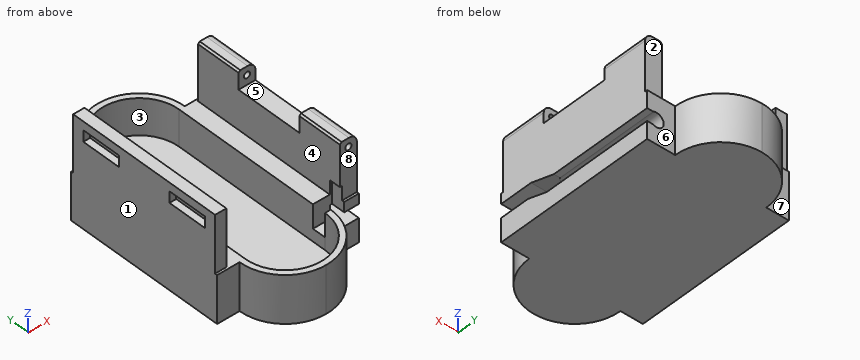
```python
from build123d import *

# Parameters (mm, degrees)
SKETCH_1_W           = 24.2
SKETCH_1_H           = 45
EXTRUDE_1_DEPTH      = 18.5
CUT_EXTRUDE_1_DEPTH  = 10.1
CUT_EXTRUDE_2_DEPTH  = 6.4
CUT_EXTRUDE_3_DEPTH  = 9.4
CUT_EXTRUDE_4_DEPTH  = 9.4
SKETCH_6_W           = 2.4
SKETCH_6_H           = 2.4
CUT_EXTRUDE_5_DEPTH  = 6.4
SKETCH_8_W           = 3.4
SKETCH_8_H           = 2.4
CUT_EXTRUDE_7_DEPTH  = 2
SKETCH_9_W           = 2.5
SKETCH_9_H           = 2
CUT_EXTRUDE_8_DEPTH  = 0.4
SKETCH_12_W          = 18.5
SKETCH_12_H          = 26.4
EXTRUDE_2_DEPTH      = 1
SKETCH_13_R          = 1.25
CUT_EXTRUDE_10_DEPTH = 26.4
SKETCH_14_W          = 2.2
SKETCH_14_H          = 26.4
CUT_EXTRUDE_11_DEPTH = 1.5
CUT_EXTRUDE_13_DEPTH = 2.95
SKETCH_19_W          = 10.1
SKETCH_19_H          = 2
EXTRUDE_3_DEPTH      = 1
SKETCH_20_W          = 1.8
SKETCH_20_H          = 2.4
EXTRUDE_4_DEPTH      = 1
SKETCH_21_W          = 1
SKETCH_21_H          = 10.1
CUT_EXTRUDE_14_DEPTH = 0.4
SKETCH_22_W          = 4.2
SKETCH_22_H          = 2.4
EXTRUDE_5_DEPTH      = 1
EXTRUDE_6_DEPTH      = 2.95
SKETCH_25_W          = 3
SKETCH_25_H          = 12
CUT_EXTRUDE_15_DEPTH = 3.2
SKETCH_26_R          = 0.55
CUT_EXTRUDE_16_DEPTH = 26
FILLET_1_R           = 1.4
SKETCH_27_W          = 2
SKETCH_27_H          = 7
CUT_EXTRUDE_17_DEPTH = 1.2
CHAMFER_1_SIZE       = 0.3


with BuildPart() as part:
    # 草图1 → 凸台-拉伸1 (new body)
    with BuildSketch(Plane.XY):
        with Locations((12.1, -22.5)):
            Rectangle(SKETCH_1_W, SKETCH_1_H)
    extrude(amount=EXTRUDE_1_DEPTH)

    # 草图2 → 切除-拉伸1 (cut)
    with BuildSketch(Plane.XY.offset(18.5)):
        Polygon((0, 0), (0, -8.5), (2, -8.5), (2, -36.5), (0, -36.5), (0, -45), (24.2, -45), (24.2, -36.5), (22.2, -36.5), (22.2, -8.5), (24.2, -8.5), (24.2, 0), align=None)
    extrude(amount=-CUT_EXTRUDE_1_DEPTH, mode=Mode.SUBTRACT)

    # 草图3 → 切除-拉伸2 (cut)
    with BuildSketch(Plane.XY.offset(8.4)):
        with BuildLine():
            Line((5, -8.1), (5, -36.9))
            ThreePointArc((5, -36.9), (12.1, -44), (19.2, -36.9))
            Line((19.2, -36.9), (19.2, -8.1))
            ThreePointArc((19.2, -8.1), (12.1, -1), (5, -8.1))
        make_face()
    extrude(amount=-CUT_EXTRUDE_2_DEPTH, mode=Mode.SUBTRACT)

    # 草图4 → 切除-拉伸3 (cut, through all)
    with BuildSketch(Plane.XY.offset(8.4)):
        with BuildLine():
            Line((4, -8.1), (0, -8.1))
            Line((0, -8.1), (0, 0))
            Line((0, 0), (12.1, 0))
            ThreePointArc((12.1, 0), (6.372435072, -2.372435072), (4, -8.1))
        make_face()
        with BuildLine():
            Line((4, -36.9), (0, -36.9))
            Line((0, -36.9), (0, -45))
            Line((0, -45), (12.1, -45))
            ThreePointArc((12.1, -45), (6.372435072, -42.627564928), (4, -36.9))
        make_face()
    extrude(amount=-CUT_EXTRUDE_3_DEPTH, mode=Mode.SUBTRACT)

    # 草图5 → 切除-拉伸4 (cut, through all)
    with BuildSketch(Plane.XY.offset(8.4)):
        with BuildLine():
            Line((20.2, -36.9), (24.2, -36.9))
            Line((24.2, -36.9), (24.2, -45))
            Line((24.2, -45), (12.1, -45))
            ThreePointArc((12.1, -45), (17.827564928, -42.627564928), (20.2, -36.9))
        make_face()
        with BuildLine():
            Line((20.2, -8.1), (24.2, -8.1))
            Line((24.2, -8.1), (24.2, 0))
            Line((24.2, 0), (12.1, 0))
            ThreePointArc((12.1, 0), (17.827564928, -2.372435072), (20.2, -8.1))
        make_face()
    extrude(amount=-CUT_EXTRUDE_4_DEPTH, mode=Mode.SUBTRACT)

    # 草图6 → 切除-拉伸5 (cut)
    with BuildSketch(Plane(origin=(24.2, 0, 0), x_dir=(0, 0, -1), z_dir=(1, 0, 0))):
        with Locations((-5.4, -35.7)):
            Rectangle(SKETCH_6_W, SKETCH_6_H)
    extrude(amount=-CUT_EXTRUDE_5_DEPTH, mode=Mode.SUBTRACT)

    # 草图8 → 切除-拉伸7 (cut)
    with BuildSketch(Plane.XY.offset(8.4)):
        with Locations((20.9, -35.7)):
            Rectangle(SKETCH_8_W, SKETCH_8_H)
    extrude(amount=-CUT_EXTRUDE_7_DEPTH, mode=Mode.SUBTRACT)

    # 草图9 → 切除-拉伸8 (cut)
    with BuildSketch(Plane.ZY.offset(-22.2)):
        with Locations((9.65, -35.5)):
            Rectangle(SKETCH_9_W, SKETCH_9_H)
    extrude(amount=-CUT_EXTRUDE_8_DEPTH, mode=Mode.SUBTRACT)

    # 草图12 → 凸台-拉伸2 (add)
    with BuildSketch(Plane(origin=(24.2, 0, 0), x_dir=(0, 0, -1), z_dir=(1, 0, 0))):
        with Locations((-9.25, -21.3)):
            Rectangle(SKETCH_12_W, SKETCH_12_H)
    extrude(amount=EXTRUDE_2_DEPTH)

    # 草图13 → 切除-拉伸10 (cut)
    with BuildSketch(Plane(origin=(0, -8.1, 0), x_dir=(1, 0, 0), z_dir=(0, 1, 0))):
        with Locations((23.5, -4.2)):
            Circle(SKETCH_13_R)
    extrude(amount=-CUT_EXTRUDE_10_DEPTH, mode=Mode.SUBTRACT)

    # 草图14 → 切除-拉伸11 (cut)
    with BuildSketch(Plane(origin=(25.2, 0, 0), x_dir=(0, 0, -1), z_dir=(1, 0, 0))):
        with Locations((-4.2, -21.3)):
            Rectangle(SKETCH_14_W, SKETCH_14_H)
    extrude(amount=-CUT_EXTRUDE_11_DEPTH, mode=Mode.SUBTRACT)

    # 草图17 → 切除-拉伸13 (cut)
    with BuildSketch(Plane(origin=(25.2, 0, 0), x_dir=(0, 0, -1), z_dir=(1, 0, 0))):
        Polygon((-6.6, -34.5), (-6.6, -31), (-5.3, -26.5), (-4.2, -26.5), (-4.2, -34.5), align=None)
    extrude(amount=-CUT_EXTRUDE_13_DEPTH, mode=Mode.SUBTRACT)

    # 草图19 → 凸台-拉伸3 (add)
    with BuildSketch(Plane(origin=(24.2, 0, 0), x_dir=(0, 0, -1), z_dir=(1, 0, 0))):
        with Locations((-13.45, -35.5)):
            Rectangle(SKETCH_19_W, SKETCH_19_H)
    extrude(amount=EXTRUDE_3_DEPTH)

    # 草图20 → 凸台-拉伸4 (add)
    with BuildSketch(Plane(origin=(24.2, 0, 0), x_dir=(0, 0, -1), z_dir=(1, 0, 0))):
        with Locations((-7.5, -35.7)):
            Rectangle(SKETCH_20_W, SKETCH_20_H)
    extrude(amount=EXTRUDE_4_DEPTH)

    # 草图21 → 切除-拉伸14 (cut)
    with BuildSketch(Plane(origin=(0, -8.1, 0), x_dir=(1, 0, 0), z_dir=(0, 1, 0))):
        with Locations((24.7, -13.45)):
            Rectangle(SKETCH_21_W, SKETCH_21_H)
    extrude(amount=-CUT_EXTRUDE_14_DEPTH, mode=Mode.SUBTRACT)

    # 草图22 → 凸台-拉伸5 (add)
    with BuildSketch(Plane(origin=(24.2, 0, 0), x_dir=(0, 0, -1), z_dir=(1, 0, 0))):
        with Locations((-2.1, -35.7)):
            Rectangle(SKETCH_22_W, SKETCH_22_H)
    extrude(amount=EXTRUDE_5_DEPTH)

    # 草图23 → 凸台-拉伸6 (add)
    with BuildSketch(Plane(origin=(22.25, 0, 0), x_dir=(0, 0, -1), z_dir=(1, 0, 0))):
        Polygon((-4.2, -34.5), (-2.4, -34.5), (-2.4, -25.5), (-4.2, -31.6), align=None)
    extrude(amount=EXTRUDE_6_DEPTH)

    # 草图25 → 切除-拉伸15 (cut)
    with BuildSketch(Plane.XY.offset(18.5)):
        with Locations((23.7, -22.5)):
            Rectangle(SKETCH_25_W, SKETCH_25_H)
    extrude(amount=-CUT_EXTRUDE_15_DEPTH, mode=Mode.SUBTRACT)

    # 草图26 → 切除-拉伸16 (cut)
    with BuildSketch(Plane.XZ.offset(36.5)):
        with Locations((23.7, 17)):
            Circle(SKETCH_26_R)
    extrude(amount=-CUT_EXTRUDE_16_DEPTH, mode=Mode.SUBTRACT)

    # 圆角1
    fillet_1_edges = [part.edges().sort_by_distance(p)[0] for p in [
        (25.2, -12.5, 18.5),
        (25.2, -32.5, 18.5),
    ]]
    fillet(fillet_1_edges, radius=FILLET_1_R)

    # 草图27 → 切除-拉伸17 (cut)
    with BuildSketch(Plane.ZY):
        with Locations((16, -14)):
            Rectangle(SKETCH_27_W, SKETCH_27_H)
        with Locations((16, -31)):
            Rectangle(SKETCH_27_W, SKETCH_27_H)
    extrude(amount=-CUT_EXTRUDE_17_DEPTH, mode=Mode.SUBTRACT)

    # 倒角1
    chamfer_1_edges = [part.edges().sort_by_distance(p)[0] for p in [
        (22.2, -32.5, 18.5),
        (22.2, -12.5, 18.5),
    ]]
    chamfer(chamfer_1_edges, length=CHAMFER_1_SIZE)


solid = part.part
```
The listing builds one solid part. Answer for the finished solid, in the listing's coordinates (mm). Face numbers are marked on the shaded views. A direction names the side the tool comes from. Round coordinates to 2 decimals unless told otherwise and drop trailing zeros. Loops run counter-clockwise (first coordinate to the right, second up) from the corner with the lowest first, then second, coordinate; pieces in that order, holes last. Notation, with made-up numbers: (-7.5, 28) - (43.5, 28) arc R21 cw to (43.5, 54) - close; hole circle Ø10 at (0.25, -24.75). An arc over 180 degrees is marked (long way). Use one line per item in the form item = value. Start each with the question number.
1. The part is cut by section A-A on z = 7.25. Determine the outline of the cut face in (x, y).
2. Consider line 1 (Z direction, x = 23.7, y = -33); line 2 (X direction, y = -9.5, z = 14); line 3 (X direction, y = -30, z = 5.5). Determine where each line is inside the solid, lowest interval first. Write a range as [from, to].
3. For a pull along Y with two mould halves and no side action, classify the marked faces 1, 2 and 3 as pulls with the +Y half, pulls with the -Y half, needs draft (parallel to the pull), parting line crosses it, or undercut.
4. The part is cut by section B-B on y = -21. Determine the outline of the cut face in (x, z), then the cut area to 3 significant figures.
5. The part is cut by section C-C on x = 21. Determine the outline of the cut face in (y, z), then the cut area to 3 significant figures.
6. The part is cut by section D-D on y = -29.5. Determine the outline of the cut face in (x, z), then the cut area to 3 significant figures.
7. A tool of negligible diameter and unlimited length cuts with its end or side. For the marked faces 4, 5, 6, 7 and 8, from which of +Z, -Z, +X, -X, +Y, -Y can it reach the whole face along a straight path? Write none if from no direction.
8. Given pin 1 Ø5 at (x, y) = (3, -14) entering from -Z; pin 2 Ø0.7 at (x, z) = (23.7, 17) entering from +Y; pin 3 Ø0.9 at (x, z) = (24, 7) entering from -Y; pin 4 Ø3 at (x, z) = (6, 8.5) entering from +Y, each flat-ended and moving along its own axis, determine where each tip first touches the part or whether it passes through.
Geometry check:
q1.outline = (0, -36.9) - (4, -36.9) arc R8.1 ccw to (20.2, -36.9) - (19.2, -36.9) arc R7.1 cw to (5, -36.9) - (5, -8.1) arc R7.1 cw to (19.2, -8.1) - (19.2, -34.5) - (22.6, -34.5) - (22.6, -36.9) - (25.2, -36.9) - (25.2, -8.1) - (20.2, -8.1) arc R8.1 ccw to (4, -8.1) - (0, -8.1) - close
q2.line_1 = [0, 4.2], [6.6, 16.45], [17.55, 18.5]
q2.line_2 = [0, 2], [22.2, 25.2]
q2.line_3 = [0, 5], [19.2, 22.25]
q3.face_1 = needs draft
q3.face_2 = pulls with the +Y half
q3.face_3 = undercut
q4.outline = (0, 0) - (25.2, 0) - (25.2, 3.1) - (24.09, 3.1) arc R1.25 cw (long way) to (24.09, 5.3) - (25.2, 5.3) - (25.2, 15.3) - (22.2, 15.3) - (22.2, 8.4) - (19.2, 8.4) - (19.2, 2) - (5, 2) - (5, 8.4) - (2, 8.4) - (2, 18.5) - (0, 18.5) - close
q4.area = 155 mm^2
q5.outline = (-36.9, 0) - (-8.1, 0) - (-8.1, 8.4) - (-34.5, 8.4) - (-34.5, 4.2) - (-36.9, 4.2) - close
q5.area = 232 mm^2
q6.outline = (0, 0) - (25.2, 0) - (25.2, 3.58) - (22.41, 3.58) arc R1.25 cw to (22.25, 4.2) - (22.25, 6.17) - (25.2, 6.17) - (25.2, 17.1) arc R1.4 ccw to (23.8, 18.5) - (22.5, 18.5) - (22.2, 18.2) - (22.2, 8.4) - (19.2, 8.4) - (19.2, 2) - (5, 2) - (5, 8.4) - (2, 8.4) - (2, 18.5) - (0, 18.5) - (0, 17) - (1.2, 17) - (1.2, 15) - (0, 15) - close; hole circle Ø1.1 at (23.7, 17)
q6.area = 160 mm^2
q7.face_4 = +Z, +Y, -Y
q7.face_5 = +Z, +X
q7.face_6 = +Z, -Z, +X, +Y
q7.face_7 = +Z, -Z, -X, +Y
q7.face_8 = +Z, +X, -X, -Y
q8.pin_1 = 0
q8.pin_2 = -8.5
q8.pin_3 = -36.9
q8.pin_4 = -1.44
